For this review, take the finished solid that the model builds, in its own axes (mm). A direction names the side the tool comes from. Coordinates: 2 decimals unless noted, no trailing zeros. Loops run counter-clockwise (first coordinate to the right, second up) from the corner with the lowest first, then second, coordinate; pieces in that order, holes last. Notation, with made-up numbers: (18, -21.75) -> (45, -21.75) arc R23 ccw to (45, 2.25) -> close; hole circle Ø2 at (53, 86.5). An arc over 180 degrees is marked (long way). Use a Markdown table: item, result.
from build123d import *

# Parameters (mm, degrees)
BOSS_EXTRUDE1_DEPTH = 27.5
SKETCH2_W           = 65
SKETCH2_H           = 4
BOSS_EXTRUDE2_DEPTH = 2
FILLET1_R           = 2
SHELL1_START        = 2
SHELL1_DEPTH        = 25.5
CUT_EXTRUDE1_REACH  = 96.24
SKETCH5_W           = 10
SKETCH5_H           = 12
BOSS_EXTRUDE3_DEPTH = 5
SKETCH7_R           = 6.5
BOSS_EXTRUDE4_DEPTH = 5
SKETCH8_R           = 4.75
SKETCH8_R_2         = 3.5
CUT_EXTRUDE2_DEPTH  = 2
SKETCH9_R           = 1.5
CUT_EXTRUDE3_DEPTH  = 95.240384125


# Read off the part's stored shape, not the designer's step: Shell1
with BuildPart() as part:
    # Sketch1 → Boss-Extrude1 (new body)
    with BuildSketch(Plane(origin=(0, 0, 0), x_dir=(1, 0, 0), z_dir=(0, 1, 0))):
        with BuildLine():
            Line((-27.5, -50), (27.5, -50))
            ThreePointArc((27.5, -50), (34.571067812, -47.071067812), (37.5, -40))
            Line((37.5, -40), (37.5, 40))
            ThreePointArc((37.5, 40), (34.571067812, 47.071067812), (27.5, 50))
            Line((27.5, 50), (-27.5, 50))
            ThreePointArc((-27.5, 50), (-34.571067812, 47.071067812), (-37.5, 40))
            Line((-37.5, 40), (-37.5, -40))
            ThreePointArc((-37.5, -40), (-34.571067812, -47.071067812), (-27.5, -50))
        make_face()
    extrude(amount=BOSS_EXTRUDE1_DEPTH)

    # Sketch2 → Boss-Extrude2 (add)
    with BuildSketch(Plane.XZ):
        with Locations((0, -40)):
            Rectangle(SKETCH2_W, SKETCH2_H)
        with Locations((0, -33.5)):
            Rectangle(SKETCH2_W, SKETCH2_H)
        with Locations((0, -27)):
            Rectangle(SKETCH2_W, SKETCH2_H)
        with Locations((0, -20.5)):
            Rectangle(SKETCH2_W, SKETCH2_H)
        with Locations((0, -14)):
            Rectangle(SKETCH2_W, SKETCH2_H)
        with Locations((0, -7.5)):
            Rectangle(SKETCH2_W, SKETCH2_H)
        with Locations((0, -1)):
            Rectangle(SKETCH2_W, SKETCH2_H)
        with Locations((0, 5.5)):
            Rectangle(SKETCH2_W, SKETCH2_H)
        with Locations((0, 12)):
            Rectangle(SKETCH2_W, SKETCH2_H)
        with Locations((0, 18.5)):
            Rectangle(SKETCH2_W, SKETCH2_H)
        with Locations((0, 25)):
            Rectangle(SKETCH2_W, SKETCH2_H)
        with Locations((0, 31.5)):
            Rectangle(SKETCH2_W, SKETCH2_H)
        with Locations((0, 38)):
            Rectangle(SKETCH2_W, SKETCH2_H)
    extrude(amount=BOSS_EXTRUDE2_DEPTH)

    # Fillet1
    fillet1_edges = [part.edges().sort_by_distance(p)[0] for p in [
        (-32.5, -2, 38),
        (0, -2, 40),
        (32.5, -2, 38),
        (0, -2, 36),
        (-32.5, -2, 31.5),
        (0, -2, 33.5),
        (32.5, -2, 31.5),
        (0, -2, 29.5),
        (-32.5, -2, 12),
        (0, -2, 14),
        (32.5, -2, 12),
        (0, -2, 10),
        (-32.5, -2, 18.5),
        (0, -2, 20.5),
        (32.5, -2, 18.5),
        (0, -2, 16.5),
        (-32.5, -2, -40),
        (0, -2, -38),
        (32.5, -2, -40),
        (0, -2, -42),
        (0, -2, -35.5),
        (-32.5, -2, -33.5),
        (0, -2, -31.5),
        (32.5, -2, -33.5),
        (-32.5, -2, -27),
        (0, -2, -25),
        (32.5, -2, -27),
        (0, -2, -29),
        (-32.5, -2, -20.5),
        (0, -2, -18.5),
        (32.5, -2, -20.5),
        (0, -2, -22.5),
        (-32.5, -2, -14),
        (0, -2, -12),
        (32.5, -2, -14),
        (0, -2, -16),
        (-32.5, -2, -7.5),
        (0, -2, -5.5),
        (32.5, -2, -7.5),
        (0, -2, -9.5),
        (-32.5, -2, -1),
        (0, -2, 1),
        (32.5, -2, -1),
        (0, -2, -3),
        (-32.5, -2, 5.5),
        (0, -2, 7.5),
        (32.5, -2, 5.5),
        (0, -2, 3.5),
        (0, -2, 23),
        (-32.5, -2, 25),
        (0, -2, 27),
        (32.5, -2, 25),
    ]]
    fillet(fillet1_edges, radius=FILLET1_R - 0.0001)  # a hair under: the kernel refuses the full size

    # Shell1 outline → Shell1 (cut)
    with BuildSketch(Plane(origin=(0, 0, 0), x_dir=(1, 0, 0), z_dir=(0, 1, 0)).offset(SHELL1_START)):
        with BuildLine():
            ThreePointArc((-35.5, -40), (-33.156854249, -45.656854249), (-27.5, -48))
            Line((-27.5, -48), (27.5, -48))
            ThreePointArc((27.5, -48), (33.156854249, -45.656854249), (35.5, -40))
            Line((35.5, -40), (35.5, 40))
            ThreePointArc((35.5, 40), (33.156854249, 45.656854249), (27.5, 48))
            Line((27.5, 48), (-27.5, 48))
            ThreePointArc((-27.5, 48), (-33.156854249, 45.656854249), (-35.5, 40))
            Line((-35.5, 40), (-35.5, -40))
        make_face()
    extrude(amount=SHELL1_DEPTH, mode=Mode.SUBTRACT)

    # Cut-Extrude1: up to this face of the body (flat: up to its plane)
    cut_extrude1_end = Plane(part.part.faces().sort_by_distance((-37.5, 13.75, 0))[0])
    # Sketch4 → Cut-Extrude1 (cut, up to the picked face)
    with BuildSketch(Plane(origin=(37.5, 0, 0), x_dir=(0, 0, -1), z_dir=(1, 0, 0)), mode=Mode.PRIVATE) as cut_extrude1_sk1:
        Polygon((40, 27.5), (-40, 27.5), (50, 13.75), (50, 27.5), align=None)
    cut_extrude1_tool1 = split(extrude(cut_extrude1_sk1.sketch, amount=-CUT_EXTRUDE1_REACH, mode=Mode.PRIVATE), bisect_by=cut_extrude1_end, keep=Keep.BOTH, mode=Mode.PRIVATE)
    add(cut_extrude1_tool1.solids().sort_by(Axis((37.5, 22.916667, -20), (-1, 0, 0)))[0], mode=Mode.SUBTRACT)

    # Sketch5 → Boss-Extrude3 (add)
    with BuildSketch(Plane(origin=(0, 2, 0), x_dir=(1, 0, 0), z_dir=(0, 1, 0))):
        with Locations((0, -32)):
            Rectangle(SKETCH5_W, SKETCH5_H)
    extrude(amount=BOSS_EXTRUDE3_DEPTH)

    # Sketch7 → Boss-Extrude4 (add)
    with BuildSketch(Plane(origin=(0, 2, 0), x_dir=(1, 0, 0), z_dir=(0, 1, 0))):
        with Locations(Location((-24.75, -21, 0), (0, 0, 270))):
            Circle(SKETCH7_R)
        with Locations(Location((24.75, -21, 0), (0, 0, 270))):
            Circle(SKETCH7_R)
    extrude(amount=BOSS_EXTRUDE4_DEPTH)

    # Sketch8 → Cut-Extrude2 (cut)
    # profile 1 of 2: a face of its own
    with BuildSketch(Plane(origin=(0, 7, 0), x_dir=(1, 0, 0), z_dir=(0, 1, 0))):
        with Locations(Location((-24.75, -21, 0), (0, 0, 270))):
            Circle(SKETCH8_R)
        with Locations(Location((-24.75, -21, 0), (0, 0, 270))):
            Circle(SKETCH8_R_2, mode=Mode.SUBTRACT)
    # profile 2 of 2: a face of its own
    with BuildSketch(Plane(origin=(0, 7, 0), x_dir=(1, 0, 0), z_dir=(0, 1, 0))):
        with Locations(Location((24.75, -21, 0), (0, 0, 270))):
            Circle(SKETCH8_R)
        with Locations(Location((24.75, -21, 0), (0, 0, 270))):
            Circle(SKETCH8_R_2, mode=Mode.SUBTRACT)
    extrude(amount=-CUT_EXTRUDE2_DEPTH, mode=Mode.SUBTRACT)

    # Sketch9 → Cut-Extrude3 (cut, through all)
    with BuildSketch(Plane(origin=(37.5, 0, 0), x_dir=(0, 0, -1), z_dir=(1, 0, 0))):
        with Locations((33, 12.5)):
            Circle(SKETCH9_R)
    extrude(amount=-CUT_EXTRUDE3_DEPTH, mode=Mode.SUBTRACT)


solid = part.part
(1) Take a section at B-B on z = 44. Write out the cut boundary in (x, y).
Found:
| item | result |
|---|---|
| outline | (-36.67, 0) -> (36.67, 0) -> (36.67, 27.5) -> (34.43, 27.5) -> (34.43, 2) -> (-34.43, 2) -> (-34.43, 27.5) -> (-36.67, 27.5) -> close |
(2) For line 1 along X through (y, z) = (6.25, 28); line 2 along X through (y, z) = (12.5, -22); line 3 along Z through (x, y) = (5, 7), list the stretches that pass through material, from the lowest coordinate up.
Found:
| item | result |
|---|---|
| line 1 | x = -37.5 to -35.5, -5 to 5, 35.5 to 37.5 |
| line 2 | x = -37.5 to -35.5, 35.5 to 37.5 |
| line 3 | z = -50 to -48, 48 to 50 |
(3) Take a section at A-A on y = 12.5. Write out the cut boundary in (x, z), plus the area to 3 significant figures.
Found:
| item | result |
|---|---|
| outline | (-37.5, -40) arc R10 ccw to (-27.5, -50) -> (27.5, -50) arc R10 ccw to (37.5, -40) -> (37.5, -34.5) -> (35.5, -34.5) -> (35.5, -40) arc R8 cw to (27.5, -48) -> (-27.5, -48) arc R8 cw to (-35.5, -40) -> (-35.5, -34.5) -> (-37.5, -34.5) -> close; (-37.5, -31.5) -> (-35.5, -31.5) -> (-35.5, 40) arc R8 cw to (-27.5, 48) -> (27.5, 48) arc R8 cw to (35.5, 40) -> (35.5, -31.5) -> (37.5, -31.5) -> (37.5, 40) arc R10 ccw to (27.5, 50) -> (-27.5, 50) arc R10 ccw to (-37.5, 40) -> close |
| area | 641 mm^2 |
(4) For pin 1 Ø21.5 at (x, z) = (8, -3.5) entering from +Y; pin 2 Ø1.5 at (x, z) = (7.5, 14) entering from -Y; pin 3 Ø2.5 at (y, z) = (12.5, -33) entering from +X, all flat-tipped, find the tip position at first contact; note any pin that passes through.
Found:
| item | result |
|---|---|
| pin 1 | stops at y = 2 |
| pin 2 | stops at y = -1.56 |
| pin 3 | passes through |
(5) Take a section at C-C on y = 23.5. Write out the cut boundary in (x, z).
Found:
| item | result |
|---|---|
| outline | (-37.5, 13.82) -> (-35.5, 13.82) -> (-35.5, 40) arc R8 cw to (-27.5, 48) -> (27.5, 48) arc R8 cw to (35.5, 40) -> (35.5, 13.82) -> (37.5, 13.82) -> (37.5, 40) arc R10 ccw to (27.5, 50) -> (-27.5, 50) arc R10 ccw to (-37.5, 40) -> close |
(6) Mouldability with a two-part tool opening along Z and no side actions: class faces 1 (the face through (32.15, -1.13, 25.03)), 2 (the face through (34.49, 13.56, 47.15)), 3 (the face through (0.46, -1.4, 17.07)) as pulls with the +Z half, pulls with the -Z half, needs draft (parallel to the pull), parting line crosses it, or undercut.
Found:
| item | result |
|---|---|
| face 1 | needs draft |
| face 2 | pulls with the +Z half |
| face 3 | undercut |
(7) For faces 4 (the face through (32.15, -1.13, 31.53)), 5 (the face through (33.219, 8.546, -45.594)), 6 (the face through (0.46, -1.4, -38.57)), list the 3-axis set-ups (+Z, -Z, +X, -X, +Y, -Y) from which the entire face can be reached by the end or side of a thin tool; tool diameter is ignored.
Found:
| item | result |
|---|---|
| face 4 | +Z, -Z, +X, -Y |
| face 5 | +Y |
| face 6 | +X, -X, -Y |
